Check sheet for the drawn part. Datum: minimum x, y, z corner. Units: mm. Give positions to 0.01 mm unless a question says otherwise; leave off trailing zeros. Order: outer loops, then holes, each group sorted by start corner. A loop starts at its lowest first (then second) coordinate and runs counter-clockwise, first axis right, second up. Notation, with made-up numbers: M -9,0 L 7,0 A24 ccw 7,34 Z; hole C 18.25,66 d3. An arc over 180 degrees is marked long. Put each result on its own line as item: value. Start each with the question number.
Q1. Mould release check, pull along Y, two halves, no side actions. Record for the marked faces 1, 2, 3 and 4: +Y half, -Y half, draft (parallel to the pull), parting line (faces both ways), or undercut.
Q2. Material ranges on L1, parallel to X at y = 7.5, z = 7; L2, parallel to X at y = 51.5, z = 1.25; L3, parallel to Y at x = 7, z = 3.25, recorded low to high.
Q3. Section check C-C on z = 0.75. Record the cut outline in (x, y), then the cut area to 3 significant figures.
Q4. Section check B-B on x = 24.75. Record the cut outline in (y, z).
Q5. Section check A-A on y = 55. Record the cut outline in (x, z).
Q6. Go/stop test with a flat-tipped pin: pin 1 (1.5 mm diameter, centred on x = 35.5, y = 42, fed in from +Z). Record where the tip stops, or that it passes through.
Q7. Section check D-D on x = 8. Record the cut outline in (y, z).
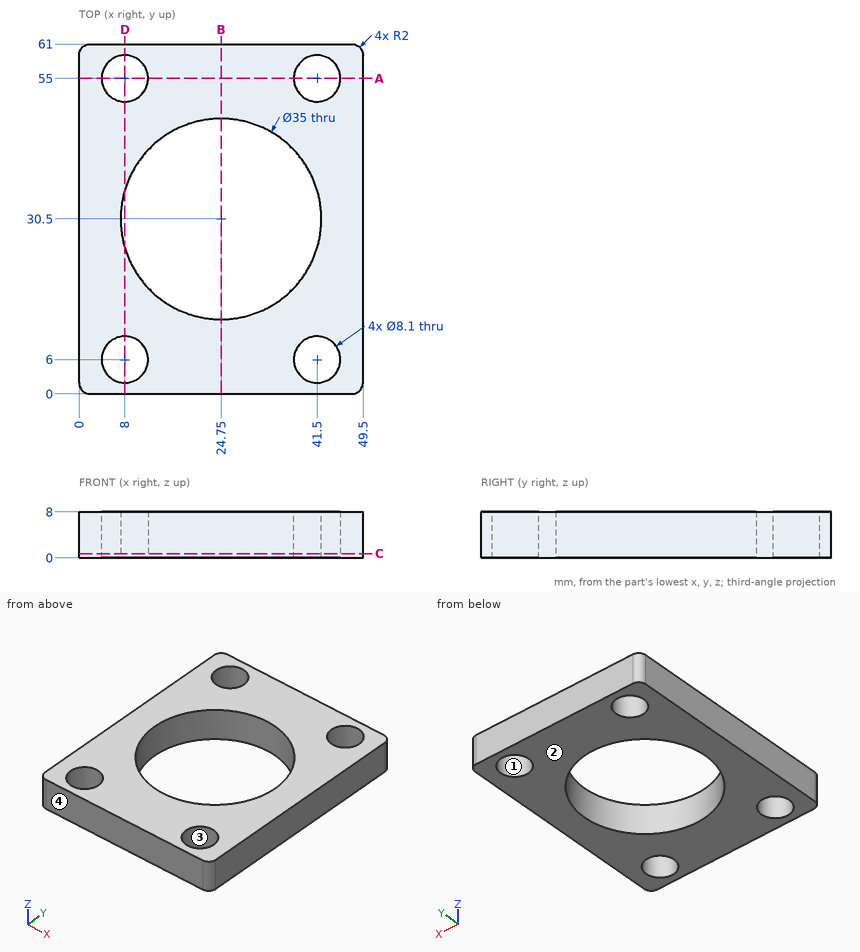
Results found:
1. face 1: undercut
1. face 2: draft
1. face 3: undercut
1. face 4: -Y half
2. L1: x = 0 to 4.24, 11.76 to 37.74, 45.26 to 49.5
2. L2: x = 0 to 5.96, 10.04 to 39.46, 43.54 to 49.5
2. L3: y = 0 to 2.08, 9.92 to 51.08, 58.92 to 61
3. outline: M 0,2 A2 ccw 2,0 L 47.5,0 A2 ccw 49.5,2 L 49.5,59 A2 ccw 47.5,61 L 2,61 A2 ccw 0,59 Z; hole C 8,6 d8.1; hole C 8,55 d8.1; hole C 24.75,30.5 d35; hole C 41.5,6 d8.1; hole C 41.5,55 d8.1
3. area: 1,850 mm^2
4. outline: M 0,0 L 13,0 L 13,8 L 0,8 Z; M 48,0 L 61,0 L 61,8 L 48,8 Z
5. outline: M 0,0 L 3.95,0 L 3.95,8 L 0,8 Z; M 12.05,0 L 37.45,0 L 37.45,8 L 12.05,8 Z; M 45.55,0 L 49.5,0 L 49.5,8 L 45.55,8 Z
6. pin 1: passes through
7. outline: M 0,0 L 1.95,0 L 1.95,8 L 0,8 Z; M 10.05,0 L 25.43,0 L 25.43,8 L 10.05,8 Z; M 35.57,0 L 50.95,0 L 50.95,8 L 35.57,8 Z; M 59.05,0 L 61,0 L 61,8 L 59.05,8 Z
